Can you work these out from the drawing? Everything is in mm from the part's minimum corner. Coordinates: 2 decimals unless noted, no trailing zeros. Order: outer loops, then holes, each group sorted by start corner. A loop starts at its lowest first (then second) coordinate and runs counter-clockwise, first axis right, second up. Notation, with made-up numbers: M 75.25,31.25 L 126.25,31.25 A25 cw 126.25,58.25 Z; hole C -13,85 d1. An arc over 180 degrees is marked long. Answer as a JSON object with one key per item and string values.
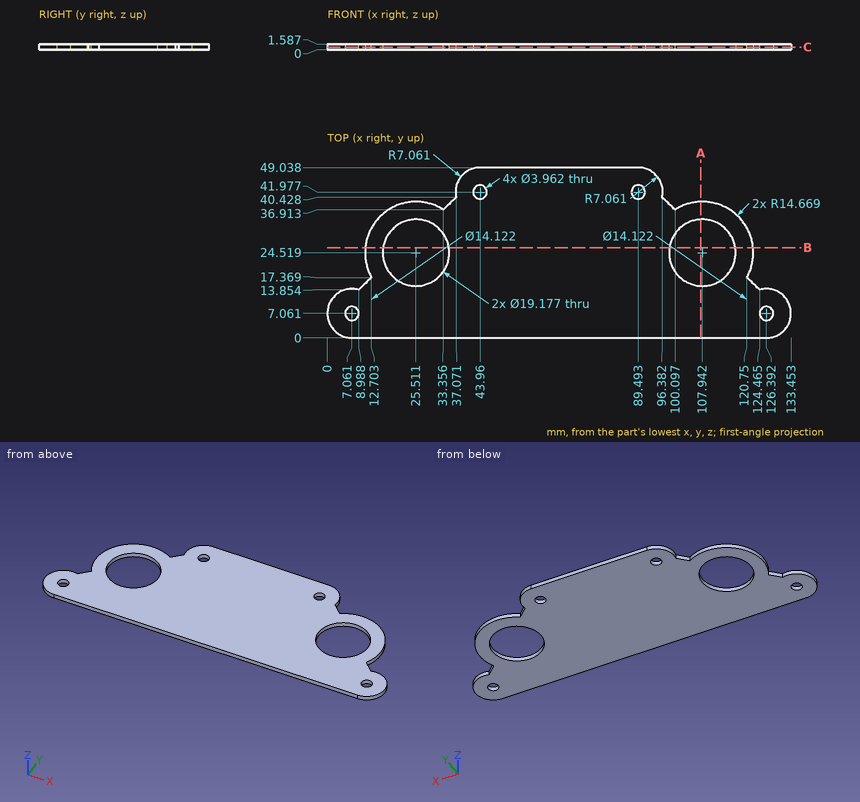
Item 1: I'm going to push a flat-ended pin straight in: pin 1 (3 mm diameter, centred on x = 100, y = 27, fed in from -Z). Where does the tip first touch, or does it pass through?
Answers follow:
{"pin 1": "stops at z = 0"}
Item 2: I want a section at A-A, the plane x = 107.5. Write out the boundary of the cut face in (y, z).
Answers follow:
{"outline": "M 0,0 L 14.94,0 L 14.94,1.59 L 0,1.59 Z; M 34.1,0 L 39.18,0 L 39.18,1.59 L 34.1,1.59 Z"}
Item 3: I want a section at C-C, the plane z = 0.7. Give the number of separate pieces and of enclosed holes in the cut face, plus the area to 3 significant figures.
Answers follow:
{"separate pieces": "1", "enclosed holes": "6", "area": "4,460 mm^2"}
Item 4: I want a section at B-B, the plane y = 26. Write out the boundary of the cut face in (x, z) (1 decimal).
Answers follow:
{"outline": "M 10.9,0 L 16,0 L 16,1.6 L 10.9,1.6 Z; M 35,0 L 98.5,0 L 98.5,1.6 L 35,1.6 Z; M 117.4,0 L 122.5,0 L 122.5,1.6 L 117.4,1.6 Z"}
Item 5: Please list where these lines run through material, in increasing order: line 1 (X direction, y = 41.5, z = 1.3) (1 decimal); line 2 (X direction, y = 26, z = 0.3) (1 decimal); line 3 (Y direction, x = 112, z = 1.05) (1 decimal).
Answers follow:
{"line 1": "x = 36.9 to 42, 45.9 to 87.6, 91.4 to 96.5", "line 2": "x = 10.9 to 16, 35 to 98.5, 117.4 to 122.5", "line 3": "y = 0 to 15.8, 33.2 to 38.6"}
